Build history of the part. All positions in model axes, mm. Face numbers are marked on the shaded views. A direction names the side the tool comes from. Give positions to 0.01 mm unless a question says otherwise; leave off trailing zeros. Loops run counter-clockwise (first coordinate to the right, second up) from the corner with the lowest first, then second, coordinate; pieces in that order, holes last. Notation, with made-up numbers: (22.25, 53.5) -> (72.25, 53.5) arc R20 cw to (72.25, 85.5) -> close; hole circle Ø4 at (87.5, -35). An arc over 180 degrees is marked (long way). Answer as a JSON object with one key per item and string values. Group by question number.
Q1. Band-saw the part on C-C, the plane y = -11.5. Write the cut outline in (x, z), plus the area to 3 significant figures.
Q2. Band-saw the part on A-A, the plane z = 18. Write the cut outline in (x, y).
Q3. Wall check: probe 1 along Y at (x, z) = (0, 27.5); probe 2 along X at (y, z) = (18, 27); probe 3 along X at (y, z) = (-28.5, 37). Give the ranges that are in metal, low to high. Write a range as from..to.
Q4. Band-saw the part on B-B, the plane x = 0. Write the cut outline in (y, z).
Q5. Tool access for the marked faces 1 and 2: list every direction of +Z, -Z, +X, -X, +Y, -Y with a clear straight run to the whole face (end or side of a thin tool).
Q6. Band-saw the part on D-D, the plane x = 50. Write the cut outline in (y, z).
Q7. Drop flat-ended pins along their axis: pin 1 (5 mm diameter, centred on y = 10.5, z = 24, fed in from +X); pin 2 (4 mm diameter, centred on x = -13, y = 31, fed in from +Z); pin 3 (3 mm diameter, centred on y = 23.5, z = 29.5, fed in from +X); pin 4 (10 mm diameter, centred on x = -27.5, y = 40, fed in from -Z). Give the stop position or say it passes through.
Q8. Two-plate mould, pull along X, no slides. Class the marked faces 3, 4 and 5: pulls with the +X half, pulls with the -X half, needs draft (parallel to the pull), parting line crosses it, or undercut.
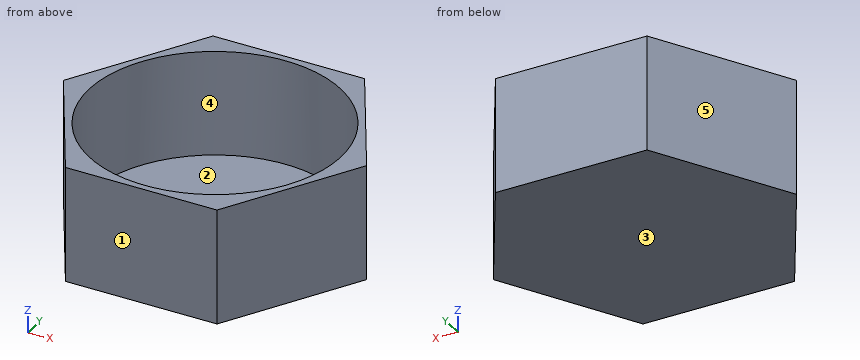
from build123d import *

# Parameters (mm, degrees)
F1_DEPTH = 4
F3_R     = 47.5
F4_DEPTH = 39.7


with BuildPart() as f1:
    # F0 (on Top) → F1 (new body)
    with BuildSketch(Plane.XY):
        Polygon((28.867513, 50), (-28.867513, 50), (-57.735027, 0), (-28.867513, -50), (28.867513, -50), (57.735027, 0), align=None)
    extrude(amount=F1_DEPTH)

    # F3 (on face) → F4 (join)
    with BuildSketch(Plane.XY.offset(4)):
        Polygon((57.735027, 0), (28.867513, 50), (-28.867513, 50), (-57.735027, 0), (-28.867513, -50), (28.867513, -50), align=None)
        Circle(F3_R, mode=Mode.SUBTRACT)
    extrude(amount=F4_DEPTH)


solid = f1.part
Worked answers:
{
 "1": {"outline": "(-51.1, 0) -> (51.1, 0) -> (51.1, 43.7) -> (46.09, 43.7) -> (46.09, 4) -> (-46.09, 4) -> (-46.09, 43.7) -> (-51.1, 43.7) -> close", "area": "806 mm2"},
 "2": {"outline": "(-57.74, 0) -> (-28.87, -50) -> (28.87, -50) -> (57.74, 0) -> (28.87, 50) -> (-28.87, 50) -> close; hole circle Ø95 at (0, 0)"},
 "3": {"probe 1": "-50..-47.5, 47.5..50", "probe 2": "-47.34..-43.96, 43.96..47.34", "probe 3": "-41.28..-38, 38..41.28"},
 "4": {"outline": "(-50, 0) -> (50, 0) -> (50, 43.7) -> (47.5, 43.7) -> (47.5, 4) -> (-47.5, 4) -> (-47.5, 43.7) -> (-50, 43.7) -> close"},
 "5": {"face 1": "+Z, -Z, +X, -X, -Y", "face 2": "+Z"},
 "6": {"outline": "(-13.4, 0) -> (13.4, 0) -> (13.4, 43.7) -> (-13.4, 43.7) -> close"},
 "7": {"pin 1": "x = 53.12", "pin 2": "z = 4", "pin 3": "x = 45.03", "pin 4": "z = 0"},
 "8": {"face 3": "needs draft", "face 4": "undercut", "face 5": "pulls with the -X half"}
}
